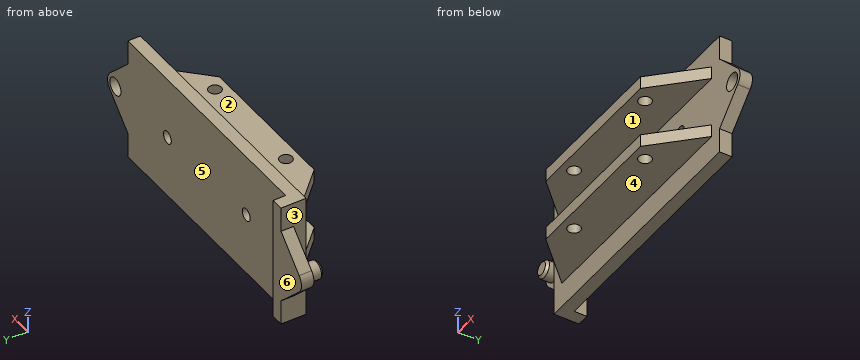
```python
from build123d import *

# Parameters (mm, degrees)
SKETCH1_R           = 3.5
BOSS_EXTRUDE1_DEPTH = 5
BOSS_EXTRUDE2_DEPTH = 5
SKETCH3_R           = 3.5
BOSS_EXTRUDE3_DEPTH = 5
SKETCH4_R           = 2.5
BOSS_EXTRUDE4_DEPTH = 15
CUT_EXTRUDE1_REACH  = 76.469
SKETCH5_W           = 100
SKETCH5_H           = 20
CUT_EXTRUDE2_REACH  = 77.8
SKETCH6_R           = 2.5
CHAMFER1_SIZE       = 1


with BuildPart() as part:
    # Sketch1 → Boss-Extrude1 (new body)
    with BuildSketch(Plane(origin=(0, 0, 0), x_dir=(1, 0, 0), z_dir=(0, 1, 0))):
        with BuildLine():
            Line((50, 15), (61.464466094, 3.535533906))
            ThreePointArc((61.464466094, 3.535533906), (62.928932188, 0), (61.464466094, -3.535533906))
            Line((61.464466094, -3.535533906), (50, -15))
            Line((50, -15), (50, -25))
            Line((50, -25), (-55, -25))
            Line((-55, -25), (-55, 25))
            Line((-55, 25), (50, 25))
            Line((50, 25), (50, 15))
        make_face()
        with Locations(Location((57.928932188, 0, 0), (0, 0, 270))):
            Circle(SKETCH1_R, mode=Mode.SUBTRACT)
    extrude(amount=BOSS_EXTRUDE1_DEPTH)

    # Sketch2 → Boss-Extrude2 (add)
    with BuildSketch(Plane(origin=(0, 5, 0), x_dir=(1, 0, 0), z_dir=(0, 1, 0))):
        with BuildLine():
            Line((-50, 25), (-50, -25))
            Line((-50, -25), (-55, -25))
            Line((-55, -25), (-55, -15))
            Line((-55, -15), (-66.464466094, -3.535533906))
            ThreePointArc((-66.464466094, -3.535533906), (-67.928932188, 0), (-66.464466094, 3.535533906))
            Line((-66.464466094, 3.535533906), (-55, 15))
            Line((-55, 15), (-55, 25))
            Line((-55, 25), (-50, 25))
        make_face()
    extrude(amount=BOSS_EXTRUDE2_DEPTH)

    # Sketch3 → Boss-Extrude3 (add)
    with BuildSketch(Plane.XZ.offset(-5)):
        with Locations(Location((-62.928932188, 0, 0), (0, 0, 270))):
            Circle(SKETCH3_R)
    extrude(amount=BOSS_EXTRUDE3_DEPTH)

    # Sketch4 → Boss-Extrude4 (add, symmetric)
    with BuildSketch(Plane.XY):
        Polygon((-50, 0), (-32.5, -17.5), (27.5, -17.5), (45, 0), align=None)
        with Locations((-22.5, -12.5)):
            Circle(SKETCH4_R, mode=Mode.SUBTRACT)
        with Locations((22.5, -12.5)):
            Circle(SKETCH4_R, mode=Mode.SUBTRACT)
    extrude(amount=BOSS_EXTRUDE4_DEPTH, both=True)

    # Sketch5 → Cut-Extrude1 (cut, up to next)
    with BuildSketch(Plane.XZ, mode=Mode.PRIVATE) as cut_extrude1_sk1:
        Rectangle(SKETCH5_W, SKETCH5_H)
    cut_extrude1_tool1 = extrude(cut_extrude1_sk1.sketch, amount=CUT_EXTRUDE1_REACH, mode=Mode.PRIVATE) & part.part
    add(cut_extrude1_tool1.solids().sort_by_distance((0, 0, 0))[0], mode=Mode.SUBTRACT)

    # Sketch6 → Cut-Extrude2 (cut, up to next)
    with BuildSketch(Plane(origin=(0, 5, 0), x_dir=(1, 0, 0), z_dir=(0, 1, 0)), mode=Mode.PRIVATE) as cut_extrude2_sk1:
        with Locations(Location((25, 0, 0), (0, 0, 270))):
            Circle(SKETCH6_R)
    cut_extrude2_tool1 = extrude(cut_extrude2_sk1.sketch, amount=-CUT_EXTRUDE2_REACH, mode=Mode.PRIVATE) & part.part
    # Sketch6 → Cut-Extrude2 (cut, up to next)
    with BuildSketch(Plane(origin=(0, 5, 0), x_dir=(1, 0, 0), z_dir=(0, 1, 0)), mode=Mode.PRIVATE) as cut_extrude2_sk2:
        with Locations(Location((-25, 0, 0), (0, 0, 270))):
            Circle(SKETCH6_R)
    cut_extrude2_tool2 = extrude(cut_extrude2_sk2.sketch, amount=-CUT_EXTRUDE2_REACH, mode=Mode.PRIVATE) & part.part
    add(cut_extrude2_tool1.solids().sort_by_distance((25, 5, 0))[0], mode=Mode.SUBTRACT)
    add(cut_extrude2_tool2.solids().sort_by_distance((-25, 5, 0))[0], mode=Mode.SUBTRACT)

    # Chamfer1
    chamfer1_edges = [part.edges().sort_by_distance(p)[0] for p in [
        (-62.928932188, 0, 3.5),
    ]]
    chamfer(chamfer1_edges, length=CHAMFER1_SIZE)


solid = part.part
```
Read the model definition and answer for the solid it produces. Units are mm, in the model's axes. Face numbers are marked on the shaded views. A direction names the side the tool comes from. Round coordinates to 2 decimals unless told otherwise and drop trailing zeros. Loops run counter-clockwise (first coordinate to the right, second up) from the corner with the lowest first, then second, coordinate; pieces in that order, holes last. Notation, with made-up numbers: (66.25, 12.5) -> (74.25, 12.5) arc R18 ccw to (74.25, 32.5) -> close; hole circle Ø2 at (-34, -20.75). An arc over 180 degrees is marked (long way). One line per item, written item: value.
1) A cutting plane is placed at C-C (x = 32). Determine the outline of the cut face in (y, z).
Answer list:
outline: (-13, -15) -> (0, -15) -> (0, -25) -> (5, -25) -> (5, 25) -> (0, 25) -> (0, 15) -> (-13, 15) -> (-13, 10) -> (0, 10) -> (0, -10) -> (-13, -10) -> close
2) For the marked faces 5 and 6, determine the directions among +Z, -Z, +X, -X, +Y, -Y from which every point of the face is accessible in a straight line to the end or side of a thin tool.
Answer list:
face 5: +Z, -Z, +X, +Y
face 6: +Z, -Z, +X, -X, +Y
3) Flat-ended cylindrical pins translate along their axes: P1, Ø6, axis at x = 10, y = -2.5, coming from the +Z side; P2, Ø4, axis at x = -58.5, z = 1.5, coming from the -Y side; P3, Ø4, axis at y = -13.5, z = 16.5, coming from the +X side; P4, Ø9, axis at x = 57.93, z = 0, coming from the +Y side. Find the tip coordinate at first contact, or state that the pin passes through.
Answer list:
P1: stops at z = 25
P2: stops at y = 0.18
P3: stops at x = 32.82
P4: stops at y = 5
4) The mould has two halves that part along Z. Classify the marked faces 1, 2, 3 and 4: pulls with the +Z half, pulls with the -Z half, needs draft (parallel to the pull), parting line crosses it, or undercut.
Answer list:
face 1: undercut
face 2: pulls with the +Z half
face 3: needs draft
face 4: pulls with the -Z half
5) A cutting plane is placed at B-B (y = -12.5). Determine the outline of the cut face in (x, z).
Answer list:
outline: (-37.5, -15) -> (-25, -15) -> (-25, -10) -> (-37.5, -10) -> close; (-37.5, 10) -> (-25, 10) -> (-25, 15) -> (-37.5, 15) -> close; (-20, -15) -> (20, -15) -> (20, -10) -> (-20, -10) -> close; (-20, 10) -> (20, 10) -> (20, 15) -> (-20, 15) -> close; (25, -15) -> (32.5, -15) -> (32.5, -10) -> (25, -10) -> close; (25, 10) -> (32.5, 10) -> (32.5, 15) -> (25, 15) -> close
6) A cutting plane is placed at D-D (z = 6.5). Determine the outline of the cut face in (x, y).
Answer list:
outline: (-63.5, 5) -> (-55, 5) -> (-55, 0) -> (58.5, 0) -> (58.5, 5) -> (-50, 5) -> (-50, 10) -> (-63.5, 10) -> close
7) Consider L1, parallel to X at y = 3.3, z = 0; L2, parallel to Z at x = -18.5, y = -2; L3, parallel to X at y = -12.5, z = 11.8. Determine where each line is inside the solid, lowest interval first. Write a range as [from, to].
Answer list:
L1: x = [-66.43, -59.43], [-55, -27.5], [-22.5, 22.5], [27.5, 54.43], [61.43, 62.93]
L2: z = [-15, -10], [10, 15]
L3: x = [-37.5, -25], [-20, 20], [25, 32.5]
8) A cutting plane is placed at A-A (y = -3.5). Determine the outline of the cut face in (x, z).
Answer list:
outline: (-46.5, -15) -> (41.5, -15) -> (41.5, -10) -> (-46.5, -10) -> close; (-46.5, 10) -> (41.5, 10) -> (41.5, 15) -> (-46.5, 15) -> close
